```python
from build123d import *

# Parameters (mm, degrees)
SKETCH1_R           = 1
BOSS_EXTRUDE1_DEPTH = 2
SKETCH2_W           = 4
SKETCH2_H           = 5
SKETCH2_W_2         = 2.463434366
SKETCH2_H_2         = 4
CUT_EXTRUDE1_DEPTH  = 1
BOSS_EXTRUDE2_DEPTH = 4
CUT_EXTRUDE2_DEPTH  = 4
CUT_EXTRUDE3_DEPTH  = 2
CUT_EXTRUDE4_START  = -3
CUT_EXTRUDE4_DEPTH  = 2.234970342


with BuildPart() as part:
    # Sketch1 → Boss-Extrude1 (new body)
    with BuildSketch(Plane.XY):
        with BuildLine():
            Line((1, 5), (1, 6))
            Line((1, 6), (2, 6))
            Line((2, 6), (2, 8))
            ThreePointArc((2, 8), (2.585786438, 9.414213562), (4, 10))
            Line((4, 10), (7, 10))
            Line((7, 10), (7, 0))
            Line((7, 0), (0, 0))
            ThreePointArc((0, 0), (-2, 2), (0, 4))
            ThreePointArc((0, 4), (0.707106781, 4.292893219), (1, 5))
        make_face()
        with Locations((0, 2)):
            Circle(SKETCH1_R, mode=Mode.SUBTRACT)
    extrude(amount=BOSS_EXTRUDE1_DEPTH)

    # Sketch2 → Cut-Extrude1 (cut)
    with BuildSketch(Plane.XY.offset(2)):
        with Locations((4, 7.5)):
            Rectangle(SKETCH2_W, SKETCH2_H)
        with Locations((-1.231717183, 2)):
            Rectangle(SKETCH2_W_2, SKETCH2_H_2)
    extrude(amount=-CUT_EXTRUDE1_DEPTH, mode=Mode.SUBTRACT)

    # Sketch3 → Boss-Extrude2 (add)
    with BuildSketch(Plane.XY.offset(2)):
        with BuildLine():
            Line((7, 10), (6, 10))
            Line((6, 10), (6, 5))
            Line((6, 5), (5, 5))
            Line((5, 5), (5, 3))
            Line((5, 3), (4, 3))
            ThreePointArc((4, 3), (1.878679656, 2.121320344), (1, 0))
            Line((1, 0), (7, 0))
            Line((7, 0), (7, 10))
        make_face()
    extrude(amount=BOSS_EXTRUDE2_DEPTH)

    # Sketch4 → Cut-Extrude2 (cut)
    with BuildSketch(Plane(origin=(7, 0, 0), x_dir=(0, 0, -1), z_dir=(1, 0, 0))):
        with BuildLine():
            Line((-3, 8), (-3, 6))
            Line((-3, 6), (-5, 4))
            Line((-5, 4), (-5, 3))
            Line((-5, 3), (-6, 3))
            Line((-6, 3), (-6, 10))
            Line((-6, 10), (-1, 10))
            ThreePointArc((-1, 10), (-2.414213562, 9.414213562), (-3, 8))
        make_face()
    extrude(amount=-CUT_EXTRUDE2_DEPTH, mode=Mode.SUBTRACT)

    # Sketch5 → Cut-Extrude3 (cut)
    with BuildSketch(Plane(origin=(0, 3, 0), x_dir=(1, 0, 0), z_dir=(0, 1, 0))):
        with BuildLine():
            Line((6, -6), (1.997304718, -6))
            Line((1.997304718, -6), (1.997304718, -4))
            Line((1.997304718, -4), (4, -4))
            ThreePointArc((4, -4), (4.585786438, -5.414213562), (6, -6))
        make_face()
    extrude(amount=-CUT_EXTRUDE3_DEPTH, mode=Mode.SUBTRACT)

    # Cut-Extrude4: read off the stored shape, not the designer's step
    # Cut-Extrude4 outline → Cut-Extrude4 (cut)
    with BuildSketch(Plane(origin=(0, 3, 0), x_dir=(1, 0, 0), z_dir=(0, 1, 0)).offset(CUT_EXTRUDE4_START)):
        with BuildLine():
            Line((1.998773483, -2.995283948), (1, -2.995283948))
            Line((1, -2.995283948), (1, -6))
            Line((1, -6), (6, -6))
            ThreePointArc((6, -6), (5.106054728, -5.78909526), (4.400646751, -5.200861851))
            Line((4.400646751, -5.200861851), (1.997304718, -4))
            Line((1.997304718, -4), (1.998773483, -2.995283948))
        make_face()
    extrude(amount=CUT_EXTRUDE4_DEPTH, mode=Mode.SUBTRACT)

    # Sketch8 → Cut-Revolve1 (revolve, cut)
    with BuildSketch(Plane(origin=(4, 0, 0), x_dir=(0, 0, -1), z_dir=(1, 0, 0)), mode=Mode.PRIVATE) as cut_revolve1_sk:
        Polygon((0, 8), (0, 8.5), (-1, 9), (-1, 8), align=None)
    revolve(cut_revolve1_sk.sketch.rotate(Axis((4, 8, -0.711012061), (0, 0, 1)), 90), axis=Axis((4, 8, -0.711012061), (0, 0, 1)), mode=Mode.SUBTRACT)


solid = part.part
```
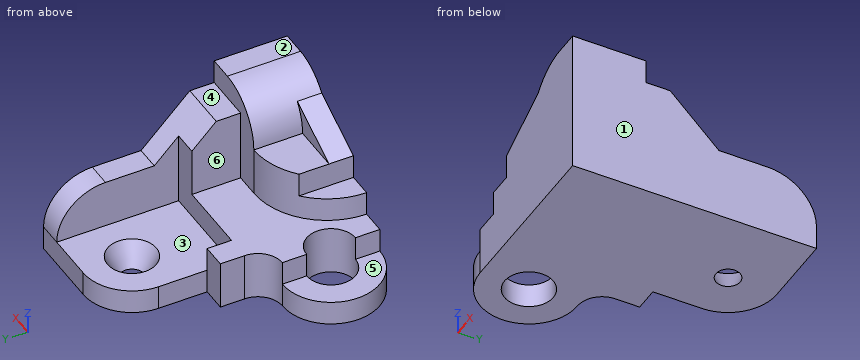
Can you work these out from the model? Positions are in its coordinate system, mm. Face numbers are marked on the shaded views. A direction names the side the tool comes from. Coordinates: 2 decimals unless noted, no trailing zeros. Loops run counter-clockwise (first coordinate to the right, second up) from the corner with the lowest first, then second, coordinate; pieces in that order, holes last. Notation, with made-up numbers: (11, 19) - (54, 19) arc R16 cw to (54, 43) - close; hole circle Ø11 at (55.5, 85). An arc over 180 degrees is marked (long way). Answer as CSV lines item,"result". Start each with the question number.
1) Suppose I cut it at A-A (y = 2.75). Please give me the cut outline in (x, z).
2) Suppose I cut it at C-C (x = -0.75). Please give me the cut outline in (y, z), plus the area to 3 significant figures.
3) Which directions (+Z, -Z, +X, -X, +Y, -Y) give clear straight access to the entire face, cutting with the end or side of a thin tool? Please do the marked faces 4, 5 and 6.
4) For pin 1 (0.9 mm diameter, centred on y = 8.5, z = 2, fed in from -X); pin 2 (1.5 mm diameter, centred on x = 3.5, z = 2, fed in from +Y); pin 3 (0.5 mm diameter, centred on x = 1.5, y = 0.5, fed in from +Z), each with a flat end and sliding along its axis, tell me the tip position at first contact or that it passes through.
5) Suppose I cut it at B-B (z = 2.5). Please give me the cut outline in (x, y), plus the area to 3 significant figures.
6) Thinking about a two-plate mould opening in X: for the marked faces 1, 2 and 3, which applies, pulls with the +X half, pulls with the -X half, needs draft (parallel to the pull), parting line crosses it, or undercut?
7) Suppose I cut it at D-D (y = 6.25). Please give me the cut outline in (x, z).
8) I need wall thicknesses on line 1 (Y direction, x = 0, z = 0.7); line 2 (X direction, y = 3.75, z = 4.95); line 3 (X direction, y = 2, z = 1.2). Which ranges of each line are inside material? Lowest first, please. Write a range as from..to.
Check result:
1,outline,"(-1.85, 0) - (-0.66, 0) - (-0.66, 1) - (-1.85, 1) - close; (0.66, 0) - (7, 0) - (7, 6) - (6, 6) arc R2 ccw to (4, 4) - (2.8, 4) - (2.8, 2) - (0.66, 2) - close"
2,outline,"(0.15, 0) - (1.34, 0) - (1.34, 1) - (0.15, 1) - close; (2.66, 0) - (3.85, 0) - (3.85, 1) - (2.66, 1) - close"
2,area,"2.39 mm²"
3,face 4,"+Z, +X, -X, +Y"
3,face 5,"+Z, -X, +Y, -Y"
3,face 6,"+Z, -X, +Y"
4,pin 1,"stops at x = 6"
4,pin 2,"stops at y = 5"
4,pin 3,"stops at z = 3"
5,outline,"(1, 0) - (7, 0) - (7, 9.32) - (6, 9.32) - (6, 5) - (5, 5) - (5, 3) - (4, 3) arc R3 ccw to start"
5,area,"24.4 mm²"
6,face 1,"pulls with the +X half"
6,face 2,"needs draft"
6,face 3,"undercut"
7,outline,"(2, 0) - (7, 0) - (7, 3) - (6, 3) - (6, 1) - (2, 1) - close"
8,line 1,"y = 0..1, 3..4"
8,line 2,"x = 5..7"
8,line 3,"x = 1..7"
